Source: CAD feature listing. Evaluate the final solid. Frame: model axes, mm. A direction names the side the tool comes from. Give positions to 0.01 mm unless a question says otherwise; leave off trailing zeros. Write each loop counter-clockwise with the first axis right and the second up, starting at its lowest first coordinate (ties: lowest second). Pieces come first, ordered by that corner, then holes. Notation, with made-up numbers: (31.25, 14) -> (66.25, 14) arc R11 cw to (66.25, 22) -> close; hole circle Ø2 at (58, -39.75). An arc over 180 degrees is marked (long way). Write item = value, one per line.
from build123d import *

# Parameters (mm, degrees)
F0_R     = 1.6
F0_W     = 3
F0_H     = 13
F1_DEPTH = 4
F2_R     = 1.25
F3_DEPTH = 25


# Not quite as in the source:
# - a feature names something its author has since deleted; it is built from what else it names


with BuildPart() as f1:
    # F0 (on Right) → F1 (new body)
    with BuildSketch(Plane.YZ):
        Polygon((-2.5, -2.5), (2.5, -2.5), (2.5, 2.5), (0.5, 2.5), (-2.5, 2.5), align=None)
        Circle(F0_R, mode=Mode.SUBTRACT)
        with Locations((-1, 9)):
            Rectangle(F0_W, F0_H)
    extrude(amount=-F1_DEPTH)

    # F2 (on face) → F3 (cut)
    with BuildSketch(Plane.XZ.offset(2.5)):
        with Locations((-2, 13)):
            Circle(F2_R)
    extrude(amount=-F3_DEPTH, mode=Mode.SUBTRACT)


solid = f1.part
1) Access query for faces 1 (the flat face through (-2, -1, 15.5)), 2 (the flat face through (-2, 2, 2.5)). Directions: +Z, -Z, +X, -X, +Y, -Y. A direction counts if a zero-diameter tool reaches every point of the face in a straight line with its end or side. Return the directions, or none.
Computed:
face_1 = +Z, +X, -X, +Y, -Y
face_2 = +Z, +X, -X, +Y
2) Material intervals for L1, parallel to Z at x = -2.75, y = 0; L2, parallel to Z at x = -2, y = -0.45; L3, parallel to Y at x = -0.9, z = 0.75, sorted ascending.
Computed:
L1 = -2.5 to -1.6, 1.6 to 12, 14 to 15.5
L2 = -2.5 to -1.54, 1.54 to 11.75, 14.25 to 15.5
L3 = -2.5 to -1.41, 1.41 to 2.5
3) Cut plane A-A (x = -3). Return the cut outline in (y, z).
Computed:
outline = (-2.5, -2.5) -> (2.5, -2.5) -> (2.5, 2.5) -> (0.5, 2.5) -> (0.5, 12.25) -> (-2.5, 12.25) -> close; (-2.5, 13.75) -> (0.5, 13.75) -> (0.5, 15.5) -> (-2.5, 15.5) -> close; hole circle Ø3.2 at (0, 0)
4) Cut plane C-C (z = 0). Return the cut outline in (x, y), then the cut area to 3 significant figures.
Computed:
outline = (-4, -2.5) -> (0, -2.5) -> (0, -1.6) -> (-4, -1.6) -> close; (-4, 1.6) -> (0, 1.6) -> (0, 2.5) -> (-4, 2.5) -> close
area = 7.20 mm²
5) Cut plane D-D (x = -2). Return the cut outline in (y, z).
Computed:
outline = (-2.5, -2.5) -> (2.5, -2.5) -> (2.5, 2.5) -> (0.5, 2.5) -> (0.5, 11.75) -> (-2.5, 11.75) -> close; (-2.5, 14.25) -> (0.5, 14.25) -> (0.5, 15.5) -> (-2.5, 15.5) -> close; hole circle Ø3.2 at (0, 0)
6) Cut plane B-B (y = 0). Return the cut outline in (x, z), then the cut area to 3 significant figures.
Computed:
outline = (-4, -2.5) -> (0, -2.5) -> (0, -1.6) -> (-4, -1.6) -> close; (-4, 1.6) -> (0, 1.6) -> (0, 15.5) -> (-4, 15.5) -> close; hole circle Ø2.5 at (-2, 13)
area = 54.3 mm²
7) Contact query for flat-ended pins moving along their axis: pin 1 (1.2 mm diameter, centred on x = -2, z = 9.5, fed in from +Y); pin 2 (2.5 mm diameter, centred on y = 0, z = 0, fed in from +X); pin 3 (1 mm diameter, centred on x = -2.5, y = 1.5, fed in from +Z). Output: stop coordinate, or through.
Computed:
pin_1 = 0.5
pin_2 = through
pin_3 = 2.5
8) Draft query along X for faces 3 (the flat face through (-4, -1, 7)), 4 (the cylindrical face through (-1.328, -1.021, 14.054)), 5 (the cylindrical face through (-1.97, -1.27, -0.97)), 6 (the flat face through (0, -1, 7)). Return one class per face: pulls with the +X half, pulls with the -X half, needs draft (parallel to the pull), parting line crosses it, or undercut.
Computed:
face_3 = pulls with the -X half
face_4 = undercut
face_5 = needs draft
face_6 = pulls with the +X half
